Work out the finished part from the listing and answer in its coordinate system (mm). Face numbers are marked on the shaded views. Give positions to 0.01 mm unless a question says otherwise; leave off trailing zeros. Order: outer loops, then holes, each group sorted by start corner. A loop starts at its lowest first (then second) coordinate and runs counter-clockwise, first axis right, second up. Notation, with made-up numbers: (-13, 38) -> (5, 38) arc R21 cw to (5, 60) -> close; hole circle Ø4 at (51, 14). An arc over 180 degrees is marked (long way). Use a Markdown table: item, result. Add a question column.
```python
from build123d import *

# Parameters (mm, degrees)
F0_W      = 6.5
F0_H      = 6.5
F1_DEPTH  = 6.5
F2_R      = 1
F3_DEPTH  = 25
F4_W      = 0.5
F4_H      = 6.5
F5_DEPTH  = 0.2
F6_W      = 6.3
F6_H      = 0.5
F7_DEPTH  = 0.2
F8_W      = 0.5
F8_H      = 6.3
F9_DEPTH  = 0.2
F10_W     = 6.1
F10_H     = 0.5
F11_DEPTH = 0.2
F12_R     = 0.3


with BuildPart() as f1:
    # F0 (on Front) → F1 (new body)
    with BuildSketch(Plane.XZ):
        with Locations((3.25, -3.25)):
            Rectangle(F0_W, F0_H)
    extrude(amount=F1_DEPTH)

    # F2 (on face) → F3 (cut)
    with BuildSketch(Plane.XZ.offset(6.5)):
        with Locations((3.25, -3.25)):
            Circle(F2_R)
    extrude(amount=-F3_DEPTH, mode=Mode.SUBTRACT)

    # F4 (on face) → F5 (cut)
    with BuildSketch(Plane.YZ.offset(6.5)):
        with Locations((-5.75, -3.25)):
            Rectangle(F4_W, F4_H)
        with Locations((-4.95, -3.25)):
            Rectangle(F4_W, F4_H)
        Polygon((-3.1, 0), (-3.1, -6.5), (-2.6, -6.5), (-2.6, -2.0569080953), (-1, -0.6072367541), (-1, -6.5), (-0.5, -6.5), (-0.5, 0), (-1, 0), (-1, -0.1072367541), (-2.6, -1.5569080953), (-2.6, 0), align=None)
    extrude(amount=-F5_DEPTH, mode=Mode.SUBTRACT)

    # F6 (on face) → F7 (cut)
    with BuildSketch(Plane.XY):
        with Locations((3.15, -5.75)):
            Rectangle(F6_W, F6_H)
        with Locations((3.15, -4.95)):
            Rectangle(F6_W, F6_H)
        Polygon((0, -2.6), (0, -3.1), (6.3, -3.1), (6.3, -2.6), (2.0569080953, -2.6), (0.6072367541, -1), (6.3, -1), (6.3, -0.5), (0, -0.5), (0, -1), (0.1072367541, -1), (1.5569080953, -2.6), align=None)
    extrude(amount=-F7_DEPTH, mode=Mode.SUBTRACT)

    # F8 (on face) → F9 (cut)
    with BuildSketch(Plane(origin=(0, 0, 0), x_dir=(0, -1, 0), z_dir=(-1, 0, 0))):
        with Locations((5.75, -3.35)):
            Rectangle(F8_W, F8_H)
        with Locations((4.95, -3.35)):
            Rectangle(F8_W, F8_H)
        Polygon((2.6, -6.5), (3.1, -6.5), (3.1, -0.2), (2.6, -0.2), (2.6, -4.3532891255), (1, -5.8029604666), (1, -0.2), (0.5, -0.2), (0.5, -6.5), (1, -6.5), (1, -6.3029604666), (2.6, -4.8532891255), align=None)
    extrude(amount=-F9_DEPTH, mode=Mode.SUBTRACT)

    # F10 (on face) → F11 (cut)
    with BuildSketch(Plane(origin=(0, 0, -6.5), x_dir=(1, 0, 0), z_dir=(0, 0, -1))):
        with Locations((3.25, 5.75)):
            Rectangle(F10_W, F10_H)
        with Locations((3.25, 4.95)):
            Rectangle(F10_W, F10_H)
        Polygon((6.3, 3.1), (0.2, 3.1), (0.2, 2.6), (4.4430919047, 2.6), (5.8927632459, 1), (0.2, 1), (0.2, 0.5), (6.3, 0.5), (6.3, 1), (6.3927632459, 1), (4.9430919047, 2.6), (6.3, 2.6), align=None)
    extrude(amount=-F11_DEPTH, mode=Mode.SUBTRACT)

    # F12
    f12_edges = [f1.edges().sort_by_distance(p)[0] for p in [
        (0, -6.25, -6.5),
        (0.2, -5.75, -6.3),
        (0.2, -4.95, -6.3),
        (0, -5.35, -6.5),
        (0, -3.9, -6.5),
        (0.2, -2.85, -6.3),
        (0, -1.8, -6.5),
        (0.2, -0.75, -6.3),
        (0, -0.25, -6.5),
        (6.5, -0.25, -6.5),
        (6.3, -0.75, -6.3),
        (6.5, -1.8, -6.5),
        (6.3, -4.95, -6.3),
        (6.5, -3.9, -6.5),
        (6.5, -5.35, -6.5),
        (6.3, -5.75, -6.3),
        (6.5, -6.25, -6.5),
        (6.5, -0.25, 0),
        (6.3, -0.75, -0.2),
        (6.5, -1.8, 0),
        (6.3, -2.85, -0.2),
        (6.5, -3.9, 0),
        (6.3, -4.95, -0.2),
        (6.5, -5.35, 0),
        (6.3, -5.75, -0.2),
        (6.5, -6.25, 0),
        (0, -0.25, 0),
        (0.2, -0.75, -0.2),
        (0, -1.8, 0),
        (0.2, -2.85, -0.2),
        (0, -3.9, 0),
        (0.2, -4.95, -0.2),
        (0, -5.35, 0),
        (0.2, -5.75, -0.2),
        (0, -6.25, 0),
        (6.3, -2.85, -6.3),
    ]]
    fillet(f12_edges, radius=F12_R)


solid = f1.part
```
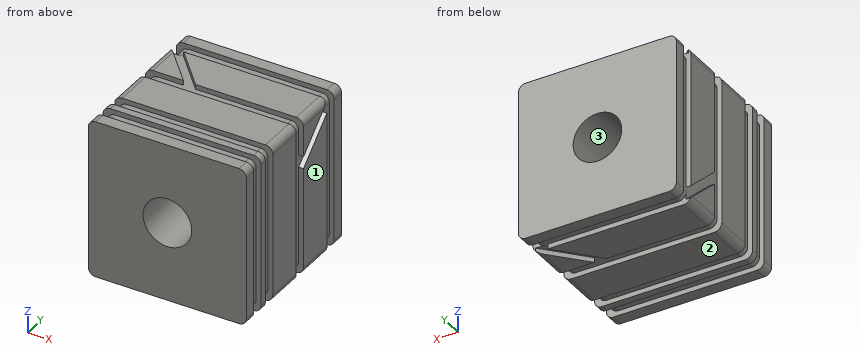
1) The part is cut by section B-B, the plane y = -1.75. Determine the outline of the cut face in (x, z), then the cut area to 3 significant figures.
2) Determine the mould class of the marked faces 1, 2 and 3 for opening direction X: released by +X, released by -X, zero draft, split by the parting line, or undercut.
3) The part is cut by section A-A, the plane y = -4.25. Determine the outline of the cut face in (x, z).
4) Straight lines are drawn through the part: line 1 (Z direction, x = 3.25, y = -4.75); line 2 (Z direction, x = 0.75, y = -5.75); line 3 (Z direction, x = 3, y = -2). For each, find the intervals that lie inside material, in ascending order.
A:
| question | item | result |
|---|---|---|
| 1 | outline | (0, -6.2) arc R0.3 ccw to (0.3, -6.5) -> (5.21, -6.5) -> (5.21, -6.3) -> (5.71, -6.3) -> (5.71, -6.5) -> (6.2, -6.5) arc R0.3 ccw to (6.5, -6.2) -> (6.5, -1.29) -> (6.3, -1.29) -> (6.3, -0.79) -> (6.5, -0.79) -> (6.5, -0.3) arc R0.3 ccw to (6.2, 0) -> (1.29, 0) -> (1.29, -0.2) -> (0.79, -0.2) -> (0.79, 0) -> (0.3, 0) arc R0.3 ccw to (0, -0.3) -> (0, -5.12) -> (0.2, -5.12) -> (0.2, -5.62) -> (0, -5.62) -> close; hole circle Ø2 at (3.25, -3.25) |
| 1 | area | 38.6 mm^2 |
| 2 | face 1 | released by +X |
| 2 | face 2 | zero draft |
| 2 | face 3 | undercut |
| 3 | outline | (0, -6.2) arc R0.3 ccw to (0.3, -6.5) -> (6.2, -6.5) arc R0.3 ccw to (6.5, -6.2) -> (6.5, -0.3) arc R0.3 ccw to (6.2, 0) -> (0.3, 0) arc R0.3 ccw to (0, -0.3) -> close; hole circle Ø2 at (3.25, -3.25) |
| 4 | line 1 | -6.3 to -4.25, -2.25 to -0.2 |
| 4 | line 2 | -6.3 to -0.2 |
| 4 | line 3 | -6.5 to -4.22, -2.28 to 0 |
